```python
from build123d import *

# Parameters (mm, degrees)
SKETCH1_W                      = 3.95
SKETCH1_H                      = 13.1
BOSS_EXTRUDE1_DEPTH            = 93
SKETCH2_W                      = 3.95
SKETCH2_H                      = 13.1
BOSS_EXTRUDE2_DEPTH            = 93
SKETCH3_W                      = 6.25
SKETCH3_H                      = 6.35
BOSS_EXTRUDE3_DEPTH            = 30
LPATTERN1_COUNT                = 4
LPATTERN1_PITCH                = 20
SKETCH4_W                      = 6.35
SKETCH4_H                      = 6.25
BOSS_EXTRUDE4_DEPTH            = 60
FILLET1_R                      = 2.5
SKETCH5_W                      = 6.25
SKETCH5_H                      = 6.25
BOSS_EXTRUDE5_DEPTH            = 25
FILLET2_R                      = 2.5
FILLET3_R                      = 2.5
SKETCH6_W                      = 6.35
SKETCH6_H                      = 6.25
BOSS_EXTRUDE6_DEPTH            = 14.35
FILLET4_R                      = 2.5
F_3_3_3_3_DIAMETER_HOLE1_D     = 3.3
F_3_3_3_3_DIAMETER_HOLE1_DEPTH = 5
F_3_3_3_3_DIAMETER_HOLE1_TIP   = 0.991420021
FILLET5_R                      = 1
FILLET6_R                      = 1


with BuildPart() as part:
    # Sketch1 → Boss-Extrude1 (new body)
    with BuildSketch(Plane(origin=(0, 0, 0), x_dir=(1, 0, 0), z_dir=(0, 1, 0))):
        with Locations((0, 6.55)):
            Rectangle(SKETCH1_W, SKETCH1_H)
    extrude(amount=BOSS_EXTRUDE1_DEPTH)



with BuildPart() as body_2:
    # Sketch2 → Boss-Extrude2 (new body)
    with BuildSketch(Plane(origin=(0, 0, 0), x_dir=(1, 0, 0), z_dir=(0, 1, 0))):
        with Locations((30, 6.55)):
            Rectangle(SKETCH2_W, SKETCH2_H)
    extrude(amount=BOSS_EXTRUDE2_DEPTH)


with BuildPart() as part_1:
    add(part.part)

    add(body_2.part)  # Boss-Extrude3 merges body 2
    # Sketch3 → Boss-Extrude3 (add)
    with BuildSketch(Plane(origin=(1.975, 0, 0), x_dir=(0, 0, -1), z_dir=(1, 0, 0))):
        with Locations((3.125, 89.825)):
            Rectangle(SKETCH3_W, SKETCH3_H)
    boss_extrude3 = extrude(amount=BOSS_EXTRUDE3_DEPTH)

    # LPattern1: Boss-Extrude3 ×4
    with Locations(*[(0, -i * LPATTERN1_PITCH, 0) for i in range(1, LPATTERN1_COUNT)]):
        add(boss_extrude3)

    # Sketch4 → Boss-Extrude4 (add)
    with BuildSketch(Plane.XZ.offset(-86.65)):
        with Locations((15, -3.125)):
            Rectangle(SKETCH4_W, SKETCH4_H)
    extrude(amount=BOSS_EXTRUDE4_DEPTH)

    # Fillet1
    fillet1_edges = [part_1.edges().sort_by_distance(p)[0] for p in [
        (18.175, 66.65, -3.125),
        (18.175, 53, -3.125),
        (18.175, 73, -3.125),
        (18.175, 86.65, -3.125),
        (18.175, 46.65, -3.125),
        (11.825, 66.65, -3.125),
        (11.825, 53, -3.125),
        (11.825, 73, -3.125),
        (11.825, 86.65, -3.125),
        (11.825, 46.65, -3.125),
        (28.025, 86.65, -3.125),
        (1.975, 86.65, -3.125),
        (28.025, 66.65, -3.125),
        (28.025, 73, -3.125),
        (1.975, 66.65, -3.125),
        (1.975, 73, -3.125),
        (28.025, 46.65, -3.125),
        (28.025, 53, -3.125),
        (1.975, 46.65, -3.125),
        (1.975, 53, -3.125),
        (28.025, 33, -3.125),
        (1.975, 33, -3.125),
        (11.825, 33, -3.125),
        (18.175, 33, -3.125),
    ]]
    fillet(fillet1_edges, radius=FILLET1_R)

    # Sketch5 → Boss-Extrude5 (add, symmetric)
    with BuildSketch(Plane.ZY.offset(-15)):
        with Locations((-3.125, 9.175)):
            Rectangle(SKETCH5_W, SKETCH5_H)
    extrude(amount=BOSS_EXTRUDE5_DEPTH, both=True)

    # Fillet2
    fillet2_edges = [part_1.edges().sort_by_distance(p)[0] for p in [
        (1.975, 12.3, -3.125),
        (28.025, 12.3, -3.125),
        (28.025, 26.65, -3.125),
        (1.975, 26.65, -3.125),
    ]]
    fillet(fillet2_edges, radius=FILLET2_R)

    # Fillet3
    fillet3_edges = [part_1.edges().sort_by_distance(p)[0] for p in [
        (31.975, 12.3, -3.125),
        (-1.975, 12.3, -3.125),
    ]]
    fillet(fillet3_edges, radius=FILLET3_R)

    # Sketch6 → Boss-Extrude6 (add)
    with BuildSketch(Plane.XZ.offset(-26.65)):
        with Locations((15, -3.125)):
            Rectangle(SKETCH6_W, SKETCH6_H)
    extrude(amount=BOSS_EXTRUDE6_DEPTH)

    # Fillet4
    fillet4_edges = [part_1.edges().sort_by_distance(p)[0] for p in [
        (18.175, 26.65, -3.125),
        (11.825, 26.65, -3.125),
        (18.175, 12.3, -3.125),
        (11.825, 12.3, -3.125),
    ]]
    fillet(fillet4_edges, radius=FILLET4_R)

    # Ø3.3 (3.3) Diameter Hole1
    with Locations(Plane.XY):
        with Locations((28.025, 49.825), (1.975, 49.825)):
            Hole(F_3_3_3_3_DIAMETER_HOLE1_D / 2, depth=F_3_3_3_3_DIAMETER_HOLE1_DEPTH)
            with Locations((0, 0, -(F_3_3_3_3_DIAMETER_HOLE1_DEPTH + F_3_3_3_3_DIAMETER_HOLE1_TIP / 2))):  # 118° drill point
                Cone(0, F_3_3_3_3_DIAMETER_HOLE1_D / 2, F_3_3_3_3_DIAMETER_HOLE1_TIP, mode=Mode.SUBTRACT)

    # Fillet5
    fillet5_edges = [part_1.edges().sort_by_distance(p)[0] for p in [
        (28.025, 0, -6.55),
        (31.975, 0, -6.55),
        (1.975, 0, -6.55),
        (-1.975, 0, -6.55),
    ]]
    fillet(fillet5_edges, radius=FILLET5_R)

    # Fillet6
    fillet6_edges = [part_1.edges().sort_by_distance(p)[0] for p in [
        (31.975, 6.05, -3.125),
        (1.975, 6.05, -3.125),
        (28.025, 6.05, -3.125),
        (-1.975, 6.05, -3.125),
    ]]
    fillet(fillet6_edges, radius=FILLET6_R)


solid = part_1.part
```
Here's how the part is built. I have some questions about the finished solid (model axes, mm). A direction names the side the tool comes from. Give positions to 0.01 mm unless a question says otherwise; leave off trailing zeros. Write each loop counter-clockwise with the first axis right and the second up, starting at its lowest first coordinate (ties: lowest second). Pieces come first, ordered by that corner, then holes. Notation, with made-up numbers: (35.25, -34) -> (53.25, -34) arc R13 cw to (53.25, -28) -> close; hole circle Ø7 at (76, 46.25). An arc over 180 degrees is marked (long way). Write each question's results on one line, items separated by ' | '.
Item 1: Suppose I cut it at C-C on x = 23.5. Write out the boundary of the cut face in (y, z), plus the area to 3 significant figures.
Output:
outline: (6.05, -6.25) -> (12.3, -6.25) -> (12.3, 0) -> (6.05, 0) -> close; (26.65, -6.25) -> (33, -6.25) -> (33, 0) -> (26.65, 0) -> close; (46.65, -6.25) -> (53, -6.25) -> (53, 0) -> (46.65, 0) -> close; (66.65, -6.25) -> (73, -6.25) -> (73, 0) -> (66.65, 0) -> close; (86.65, -6.25) -> (93, -6.25) -> (93, 0) -> (86.65, 0) -> close | area: 198 mm^2
Item 2: Suppose I cut it at B-B on y = 58.5. Write out the boundary of the cut face in (x, z) (3 decimals), plus the area to 3 significant figures.
Output:
outline: (-1.975, -13.1) -> (1.975, -13.1) -> (1.975, 0) -> (-1.975, 0) -> close; (11.825, -6.25) -> (18.175, -6.25) -> (18.175, 0) -> (11.825, 0) -> close; (28.025, -13.1) -> (31.975, -13.1) -> (31.975, 0) -> (28.025, 0) -> close | area: 143 mm^2
Item 3: If I drill on L1, parallel to Y at x = 5.5, z = -0.5; L2, parallel to X at y = 37, z = -3.5 (3 decimals); L3, parallel to X at y = 18, z = -7.75 (3 decimals), over which ranges is the centre line in solid material (lowest first)?
Output:
L1: y = 6.05 to 12.3, 26.65 to 33, 46.65 to 53, 66.65 to 73, 86.65 to 93 | L2: x = -1.975 to 1.975, 11.825 to 18.175, 28.025 to 31.975 | L3: x = -1.975 to 1.975, 28.025 to 31.975
Item 4: For pin 1 Ø2 at (x, y) = (4.5, 30) entering from +Z; pin 2 Ø1.5 at (x, z) = (19, -3.5) entering from -Y; pin 3 Ø2 at (x, y) = (14.5, 69.5) entering from -Z; pin 4 Ø7 at (x, z) = (35, -3.5) entering from -Y, each with a flat end and sliding along its axis, tell me the tip position at first contact or that it passes through.
Output:
pin 1: stops at z = 0 | pin 2: stops at y = 6.05 | pin 3: stops at z = -6.25 | pin 4: stops at y = 0.15
Item 5: We'd pull the mould along X, two halves only. Please class faces 1 (the face through (18.89, 53.75, -3.08)), 2 (the face through (17, 46, 0)): pulls with the +X half, pulls with the -X half, needs draft (parallel to the pull), parting line crosses it, or undercut.
Output:
face 1: undercut | face 2: needs draft
Item 6: On a 3-axis mill with a long thin cutter (end or side, diameter ignored), from which of +Z, -Z, +X, -X, +Y, -Y can I reach the whole of each face in a straight line? I mean faces 3 (the face through (15, 6.05, -3)), 4 (the face through (27.27, 65.94, -3.17)), 5 (the face through (15, 93, -4)). Say none if no direction works.
Output:
face 3: +Z, -Z, -Y | face 4: +Z, -Z | face 5: +Z, -Z, +X, -X, +Y
Item 7: Suppose I cut it at A-A on z = -10.75. Write out the boundary of the cut face in (x, y) (3 decimals), plus the area to 3 significant figures.
Output:
outline: (-1.975, 1) arc R1 ccw to (-0.975, 0) -> (0.975, 0) arc R1 ccw to (1.975, 1) -> (1.975, 93) -> (-1.975, 93) -> close; (28.025, 1) arc R1 ccw to (29.025, 0) -> (30.975, 0) arc R1 ccw to (31.975, 1) -> (31.975, 93) -> (28.025, 93) -> close | area: 734 mm^2
Item 8: Suppose I cut it at D-D on y = 29. Write out the boundary of the cut face in (x, z) (3 decimals).
Output:
outline: (-1.975, -13.1) -> (1.975, -13.1) -> (1.975, -6.25) -> (28.025, -6.25) -> (28.025, -13.1) -> (31.975, -13.1) -> (31.975, 0) -> (-1.975, 0) -> close
